Input: part model. Units: mm. Frame: model coordinates. A direction names the side the tool comes from. Round coordinates to 2 decimals unless told otherwise and drop trailing zeros. Loops run counter-clockwise (first coordinate to the right, second up) from the corner with the lowest first, then second, coordinate; pieces in that order, holes last. Notation, with made-up numbers: (2, -2.75) - (13, -2.75) arc R20 ccw to (13, 23.25) - close; hole circle Ø2 at (16, 1.5). An arc over 180 degrees is marked (long way). Use CSV: the item, a comma, the result in double quotes. Start each with the question number.
1. Pull-direction query (Z, two-part tool) for faces 1 (the cylindrical face through (12, 9.1, -8.8)), 2 (the flat face through (7, 0, -9)), 3 (the flat face through (5, 2.5, -10)), 4 (the flat face through (10, 0, 11)); classes: +Z half, -Z half, draft (parallel to the pull), parting line (faces both ways), or undercut.
2. Cut plane C-C (z = 5.25). Give the number of separate pieces and of enclosed holes in the cut face, and give its area (3 significant figures).
3. Cut plane B-B (y = 12.5). Return loops of the section in (x, z).
4. Material intervals for probe 1 along X at (y, z) = (0, 10.45); probe 2 along Y at (x, z) = (17.5, -10.35); probe 3 along Z at (x, y) = (11, -1.25), sorted ascending. Write a range as from..to.
5. Pin query (flat end, axial travel): P1, Ø0.6, axis at x = 0.5, y = 12.5, coming from the -Z side; P2, Ø8, axis at x = -4.5, z = -3.5, coming from the -Y side; P3, Ø6, axis at x = -20.5, y = 10.5, coming from the -Z side; P4, Ø1.9, axis at y = -4.5, z = -5, coming from the -X side. Return the tip coordinate at first contact, or that it passes through.
6. Access query for faces 5 (the flat face through (12, -7.2, -0.1)), 6 (the cylindrical face through (-20.07, 11.14, -6.81)), 7 (the cylindrical face through (-20.07, 10.16, 5.31)), 8 (the cylindrical face through (11.958, 9.212, 8.714)), 9 (the flat face through (-5, 7.995, -9)). Directions: +Z, -Z, +X, -X, +Y, -Y. A direction counts if a zero-diameter tool reaches every point of the face in a straight line with its end or side. Return the directions, or none.
7. Cut plane A-A (x = -9). Return loops of the section in (y, z), and give its area (3 significant figures).
8. Cut plane D-D (x = -36). Return loops of the section in (y, z).
```python
from build123d import *

# Parameters (mm, degrees)
SKETCH1_W                = 2
SKETCH1_H                = 5
BOSS_EXTRUDE1_DEPTH      = 15
BOSS_EXTRUDE1_2_DEPTH    = 15
SKETCH2_W                = 1
SKETCH2_H                = 5
BOSS_EXTRUDE2_DEPTH      = 5
CUT_EXTRUDE1_DEPTH       = 30.107559156
CUT_EXTRUDE1_DEPTH_BACK  = 30.107559156
SKETCH3_R                = 1.5
SWEEP1_START             = 9
SWEEP1_DEPTH             = 6
BOSS_EXTRUDE3_DEPTH      = 12
CUT_EXTRUDE2_DEPTH       = 5
FILLET1_R                = 2
BOSS_EXTRUDE6_START      = -6
SKETCH7_W                = 6
SKETCH7_H                = 2
BOSS_EXTRUDE6_DEPTH      = 51
BOSS_EXTRUDE7_DEPTH      = 3
BOSS_EXTRUDE7_DEPTH_BACK = 9
SKETCH8_R                = 1.5
FILLET2_R                = 2.5
BOSS_EXTRUDE10_DEPTH     = 10
LPATTERN1_COUNT          = 2
LPATTERN1_PITCH          = 15


# Read off the part's stored shape, not the designer's step: Sweep1
with BuildPart() as part:
    # Sketch1 → Boss-Extrude1 (new body)
    with BuildSketch(Plane(origin=(0, 0, 0), x_dir=(0, 0, -1), z_dir=(1, 0, 0))):
        with Locations((-10, 0)):
            Rectangle(SKETCH1_W, SKETCH1_H)
    extrude(amount=BOSS_EXTRUDE1_DEPTH)



with BuildPart() as body_2:
    # Sketch1 → Boss-Extrude1 2 (new body)
    with BuildSketch(Plane(origin=(0, 0, 0), x_dir=(0, 0, -1), z_dir=(1, 0, 0))):
        with Locations((10, 0)):
            Rectangle(SKETCH1_W, SKETCH1_H)
    extrude(amount=BOSS_EXTRUDE1_2_DEPTH)


with BuildPart() as part_1:
    add(part.part)

    add(body_2.part)  # Boss-Extrude2 merges body 2
    # Sketch2 → Boss-Extrude2 (add)
    with BuildSketch(Plane(origin=(15, 0, 0), x_dir=(0, 0, -1), z_dir=(1, 0, 0))):
        with Locations((10.5, 0)):
            Rectangle(SKETCH2_W, SKETCH2_H)
        with Locations((-10.5, 0)):
            Rectangle(SKETCH2_W, SKETCH2_H)
    extrude(amount=BOSS_EXTRUDE2_DEPTH)

    # Sketch3 → Cut-Extrude1 (cut, two sides: drawn at the far end of the back side and taken through both)
    with BuildSketch(Plane.XY.offset(-10).offset(-CUT_EXTRUDE1_DEPTH_BACK)):
        with Locations((17.5, 0)):
            Circle(SKETCH3_R)
    extrude(amount=CUT_EXTRUDE1_DEPTH + CUT_EXTRUDE1_DEPTH_BACK, mode=Mode.SUBTRACT)

    # Sweep1 outline → Sweep1 (add)
    with BuildSketch(Plane.YZ.offset(SWEEP1_START)):
        with BuildLine():
            ThreePointArc((2.5, -11), (13.5, 0), (2.5, 11))
            Line((2.5, 11), (2.5, 9))
            ThreePointArc((2.5, 9), (11.5, 0), (2.5, -9))
            Line((2.5, -9), (2.5, -11))
        make_face()
    extrude(amount=SWEEP1_DEPTH)

    # Sketch5 → Boss-Extrude3 (add)
    with BuildSketch(Plane(origin=(0, 0, 0), x_dir=(0, 0, -1), z_dir=(1, 0, 0))):
        with BuildLine():
            Line((-9, -2.5), (-11, -2.5))
            add(Edge.make_bspline(
                [(-11, -2.5), (-11, -8.980170496), (0, -8.980170496)],
                knots=[3.141592654, 3.141592654, 3.141592654, 4.71238898, 4.71238898, 4.71238898], degree=2, weights=[1, 0.707106781, 1]))
            Line((0, -8.980170496), (0, -7.009343108))
            add(Edge.make_bspline(
                [(-9, -2.5), (-9, -7.009343108), (0, -7.009343108)],
                knots=[3.141592654, 3.141592654, 3.141592654, 4.71238898, 4.71238898, 4.71238898], degree=2, weights=[1, 0.707106781, 1]))
        make_face()
    boss_extrude3 = extrude(amount=BOSS_EXTRUDE3_DEPTH)

    # Sketch6 → Cut-Extrude2 (cut)
    with BuildSketch(Plane.ZY):
        with BuildLine():
            Line((11, -2.5), (9, -2.5))
            add(Edge.make_bspline(
                [(0, -7.009343108), (9, -7.009343108), (9, -2.5)],
                knots=[4.71238898, 4.71238898, 4.71238898, 6.283185307, 6.283185307, 6.283185307], degree=2, weights=[1, 0.707106781, 1]))
            Line((0, -7.009343108), (0, -8.980170496))
            add(Edge.make_bspline(
                [(0, -8.980170496), (11, -8.980170496), (11, -2.5)],
                knots=[4.71238898, 4.71238898, 4.71238898, 6.283185307, 6.283185307, 6.283185307], degree=2, weights=[1, 0.707106781, 1]))
        make_face()
    cut_extrude2 = extrude(amount=-CUT_EXTRUDE2_DEPTH, mode=Mode.SUBTRACT)

    # Mirror2: Boss-Extrude3, Cut-Extrude2 across plane
    add(boss_extrude3.mirror(Plane(origin=(12, -8.980170496, 0), x_dir=(1, 0, 0), z_dir=(0, 0, 1))))
    add(cut_extrude2.mirror(Plane(origin=(12, -8.980170496, 0), x_dir=(1, 0, 0), z_dir=(0, 0, 1))), mode=Mode.SUBTRACT)

    # Fillet1
    fillet1_edges = [part_1.edges().sort_by_distance(p)[0] for p in [
        (0, -2.5, -10),
        (0, 2.5, -10),
        (0, 2.5, 10),
        (0, -2.5, 10),
    ]]
    fillet(fillet1_edges, radius=FILLET1_R)

    # Sketch7 → Boss-Extrude6 (add)
    with BuildSketch(Plane.ZY.offset(-9).offset(BOSS_EXTRUDE6_START)):
        with Locations((0, 12.5)):
            Rectangle(SKETCH7_W, SKETCH7_H)
    extrude(amount=BOSS_EXTRUDE6_DEPTH)

    # Sketch8 → Boss-Extrude7 (add, two sides: drawn at the far end of the back side and taken through both)
    with BuildSketch(Plane.XY.offset(3).offset(-BOSS_EXTRUDE7_DEPTH_BACK)):
        with Locations((-36, 12.5)):
            Circle(SKETCH8_R)
    extrude(amount=BOSS_EXTRUDE7_DEPTH + BOSS_EXTRUDE7_DEPTH_BACK)

    # Fillet2
    fillet2_edges = [part_1.edges().sort_by_distance(p)[0] for p in [
        (20, -2.5, -10.5),
        (20, -2.5, 10.5),
    ]]
    fillet(fillet2_edges, radius=FILLET2_R)

    # 3DSketch3 → Boss-Extrude10 (add)
    with BuildSketch(Plane(origin=(-10, 7.995255445, 9.529017137), x_dir=(0, 0, -1), z_dir=(1, 0, 0))):
        with BuildLine():
            Line((0, 0), (2, 0))
            ThreePointArc((2, 0), (9.529017137, 3.825899604), (17.058034273, 0))
            Line((17.058034273, 0), (19.058034273, 0))
            ThreePointArc((19.058034273, 0), (15.031388903, 4.029654263), (9.529017137, 5.504744555))
            ThreePointArc((9.529017137, 5.504744555), (4.026645371, 4.029654263), (0, 0))
        make_face()
    boss_extrude10 = extrude(amount=BOSS_EXTRUDE10_DEPTH)

    # LPattern1: Boss-Extrude10 ×2
    with Locations(*[(-i * LPATTERN1_PITCH, 0, 0) for i in range(1, LPATTERN1_COUNT)]):
        add(boss_extrude10)


solid = part_1.part
```
Established:
1,face 1,"-Z half"
1,face 2,"undercut"
1,face 3,"draft"
1,face 4,"+Z half"
2,separate pieces,"5"
2,enclosed holes,"0"
2,area,"74.7 mm2"
3,outline,"(-37.5, -6) - (-34.5, -6) - (-34.5, -3) - (-25, -3) - (-25, -4.58) - (-15, -4.58) - (-15, -3) - (-10, -3) - (-10, -4.58) - (0, -4.58) - (0, -3) - (9, -3) - (9, -4.58) - (15, -4.58) - (15, 4.58) - (9, 4.58) - (9, 3) - (0, 3) - (0, 4.58) - (-10, 4.58) - (-10, 3) - (-15, 3) - (-15, 4.58) - (-25, 4.58) - (-25, 3) - (-34.5, 3) - (-34.5, 6) - (-37.5, 6) - close"
4,probe 1,"x = 0..16, 19..20"
4,probe 2,"y = -2.5..-1.5, 1.5..2.5"
4,probe 3,"z = -11..-9, 9..11"
5,P1,"stops at z = -3"
5,P2,"stops at y = 8.03"
5,P3,"stops at z = -9.53"
5,P4,"passes through"
6,face 5,"+Z, -Z, +X, -Y"
6,face 6,"-Z, +X, +Y"
6,face 7,"-Y"
6,face 8,"+Z, +X, +Y"
6,face 9,"+Z, -Z, -X, -Y"
7,outline,"(8, -9.53) arc R11 ccw to (13.08, -3) - (13.5, -3) - (13.5, 3) - (13.08, 3) arc R11 ccw to (8, 9.53) - (8, 7.53) arc R9.32 cw to (11.5, 2.43) - (11.5, -2.43) arc R9.32 cw to (8, -7.53) - close"
7,area,"36.0 mm2"
8,outline,"(11, -6) - (14, -6) - (14, 6) - (11, 6) - close"
